Solid Edge part; units mm, degrees
sketch "Sketch1" plane through (0, 0, 0) normal (0, -1, 0) x (1, 0, 0)
  circle A0 centre (0, 0) radius 4.5
extrude "Protrusion1" add sketch "Sketch1" along normal blind 1
sketch "Sketch2" plane through (0, 0, 0) normal (0, -1, 0) x (1, 0, 0)
  circle A0 centre (0, 0) radius 3
extrude "Extrusionsausprägung_2" add sketch "Sketch2" along normal blind 7
sketch "Sketch3" plane through (0, 0, 0) normal (0, -1, 0) x (1, 0, 0)
  circle A0 centre (0, 0) radius 2
extrude "Cutout1" cut sketch "Sketch3" along normal through all
Build history of the part. All positions in model axes, mm. Give positions to 0.01 mm unless a question says otherwise; leave off trailing zeros. Loops run counter-clockwise (first coordinate to the right, second up) from the corner with the lowest first, then second, coordinate; pieces in that order, holes last.
Item 1: Slice it at D-D, the plane x = 4. List the corners of the cut face in (y, z), and give its area (3 significant figures).
Answers follow:
outline: (-1, -2.06) - (0, -2.06) - (0, 2.06) - (-1, 2.06) - close
area: 4.12 mm2
Item 2: Flat gauge pins, fed straight in: pin 1 (1 mm diameter, centred on x = 3.5, z = -2.5, fed in from -Y); pin 2 (3 mm diameter, centred on y = -4, z = -2.5, fed in from -X); pin 3 (2 mm diameter, centred on y = -2.5, z = 2.5, fed in from -X). Where does each tip first touch, or does it go through?
Answers follow:
pin 1: stops at y = -1
pin 2: stops at x = -2.83
pin 3: stops at x = -2.6
Item 3: Slice it at B-B, the plane x = 0. List the corners of the cut face in (y, z).
Answers follow:
outline: (-7, -3) - (-1, -3) - (-1, -4.5) - (0, -4.5) - (0, -2) - (-7, -2) - close; (-7, 2) - (0, 2) - (0, 4.5) - (-1, 4.5) - (-1, 3) - (-7, 3) - close
Item 4: Slice it at A-A, the plane z = 0. List the corners of the cut face in (x, y).
Answers follow:
outline: (-4.5, -1) - (-3, -1) - (-3, -7) - (-2, -7) - (-2, 0) - (-4.5, 0) - close; (2, -7) - (3, -7) - (3, -1) - (4.5, -1) - (4.5, 0) - (2, 0) - close
Item 5: Slice it at C-C, the plane y = -4.5. List the corners of the cut face in (x, z), and give its area (3 significant figures).
Answers follow:
outline: circle Ø6 at (0, 0); hole circle Ø4 at (0, 0)
area: 15.7 mm2
Item 6: Pull direction X, two halves, no side cores. Call faces 1 (the face through (-3, -4, 0)), 2 (the face through (0, -3, 2)), 3 (the face through (-3, -1, -1)): released by +X, released by -X, zero draft, split by the parting line, or undercut.
Answers follow:
face 1: split by the parting line
face 2: undercut
face 3: zero draft
Item 7: Drill centre lines: line 1 (X direction, y = -5, z = 0); line 2 (Z direction, x = -1.5, y = -6.25). Where is each one in solid material? Low to high.
Answers follow:
line 1: x = -3 to -2, 2 to 3
line 2: z = -2.6 to -1.32, 1.32 to 2.6
